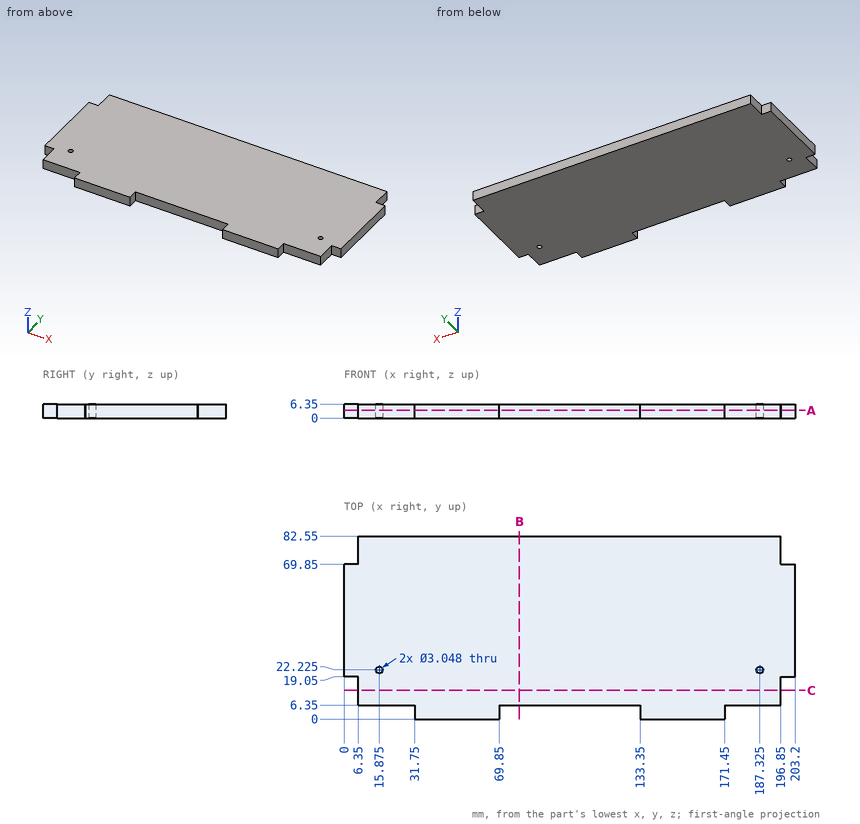
Design review of the part shown in the three views and the two pictorial views. Dimensions are in mm from the part's minimum x, y and z. Give positions to 0.01 mm unless a question says otherwise; leave off trailing zeros. Loops run counter-clockwise (first coordinate to the right, second up) from the corner with the lowest first, then second, coordinate; pieces in that order, holes last. Notation, with made-up numbers: (76, 75.25) - (120, 75.25) arc R13 ccw to (120, 82.25) - close; hole circle Ø4 at (23.25, 23). An arc over 180 degrees is marked (long way). Use CSV: the item, a comma, the result in double quotes. Start each with the question number.
1. Add section C-C (y = 13). State the section outline as (x, z) points, plus the area to 3 significant figures.
2. Wall thickness on L1, parallel to X at y = 5, z = 2; L2, parallel to X at y = 76.5, z = 0.75; L3, parallel to Y at x = 101.5, z = 2: over which ranges is each line inside the solid? List them lowest first.
3. Add section B-B (x = 79). State the section outline as (y, z) points.
4. Add section A-A (z = 3.5). State the section outline as (x, y) points (3 decimals), plus the area to 3 significant figures.
5. Insertion check: P1, Ø3, axis at y = 16.5, z = 5.5, coming from the -X side; P2, Ø3, axis at y = 11, z = 2, coming from the +X side; P3, Ø1.9, axis at y = 3, z = 2, coming from the -X side; P4, Ø1.8, axis at x = 187.325, y = 22.225, coming from the +Z side. Each pin has a flat end and moves straight along its axis. Give the tip position at first contact, or say it passes through.
Results found:
1,outline,"(6.35, 0) - (196.85, 0) - (196.85, 6.35) - (6.35, 6.35) - close"
1,area,"1,210 mm²"
2,L1,"x = 31.75 to 69.85, 133.35 to 171.45"
2,L2,"x = 6.35 to 196.85"
2,L3,"y = 6.35 to 82.55"
3,outline,"(6.35, 0) - (82.55, 0) - (82.55, 6.35) - (6.35, 6.35) - close"
4,outline,"(0, 19.05) - (6.35, 19.05) - (6.35, 6.35) - (31.75, 6.35) - (31.75, 0) - (69.85, 0) - (69.85, 6.35) - (133.35, 6.35) - (133.35, 0) - (171.45, 0) - (171.45, 6.35) - (196.85, 6.35) - (196.85, 19.05) - (203.2, 19.05) - (203.2, 69.85) - (196.85, 69.85) - (196.85, 82.55) - (6.35, 82.55) - (6.35, 69.85) - (0, 69.85) - close; hole circle Ø3.048 at (15.875, 22.225); hole circle Ø3.048 at (187.325, 22.225)"
4,area,"15,600 mm²"
5,P1,"stops at x = 6.35"
5,P2,"stops at x = 196.85"
5,P3,"stops at x = 31.75"
5,P4,"passes through"
